The figure shows three views and two pictorial views of one solid part (mm, origin at its lowest corner). Answer the questions. A direction names the side the tool comes from. Coordinates: 2 decimals unless noted, no trailing zeros. Loops run counter-clockwise (first coordinate to the right, second up) from the corner with the lowest first, then second, coordinate; pieces in that order, holes last. Notation, with made-up numbers: (19, 3.25) - (51, 3.25) arc R28 ccw to (51, 34.25) - close; hole circle Ø7 at (35, 26.25). An arc over 180 degrees is marked (long way). One line per question, with ' | ' between items.
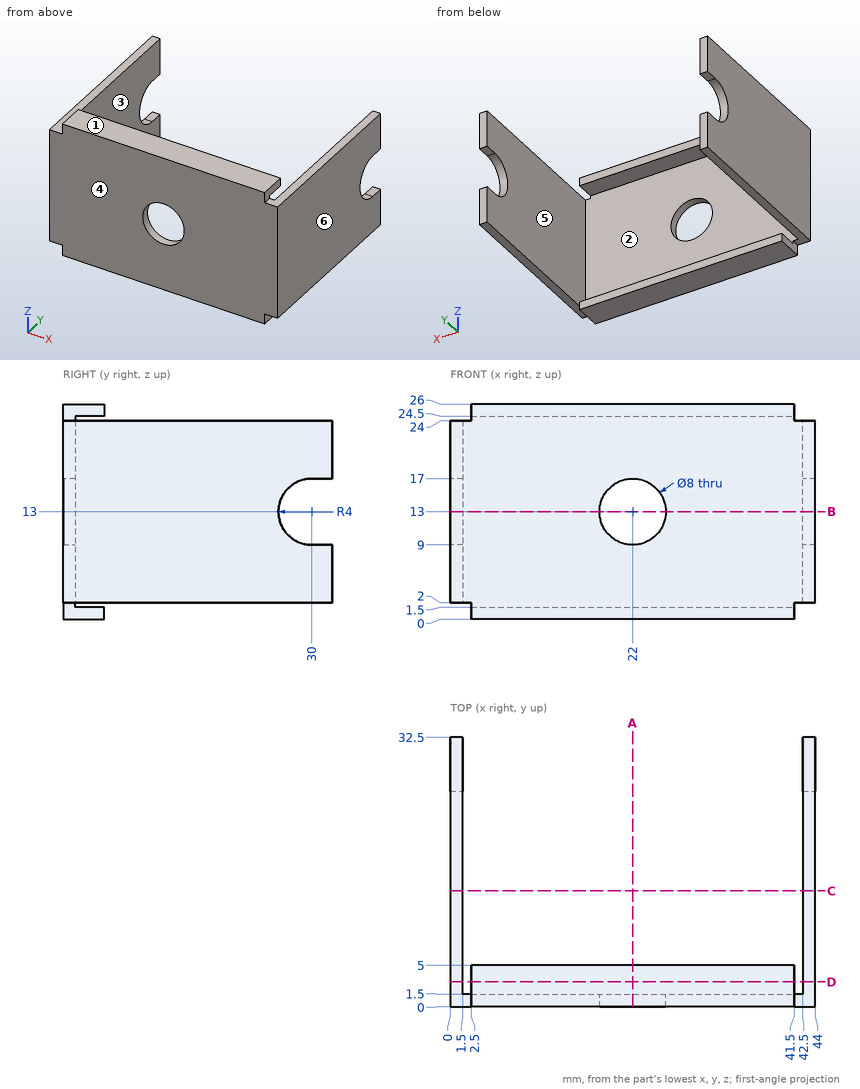
Item 1: Find section D-D, the plane y = 3. Write down the section's boundary in (x, z), plus the area to 3 significant figures.
Taken from the geometry:
outline: (0, 2) - (1.5, 2) - (1.5, 24) - (0, 24) - close; (2.5, 0) - (41.5, 0) - (41.5, 1.5) - (2.5, 1.5) - close; (2.5, 24.5) - (41.5, 24.5) - (41.5, 26) - (2.5, 26) - close; (42.5, 2) - (44, 2) - (44, 24) - (42.5, 24) - close | area: 183 mm2
Item 2: Find section C-C, the plane y = 14. Write down the section's boundary in (x, z).
Taken from the geometry:
outline: (0, 2) - (1.5, 2) - (1.5, 24) - (0, 24) - close; (42.5, 2) - (44, 2) - (44, 24) - (42.5, 24) - close
Item 3: Find section B-B, the plane z = 13. Write down the section's boundary in (x, y), plus the area to 4 significant figures.
Taken from the geometry:
outline: (0, 0) - (18, 0) - (18, 1.5) - (1.5, 1.5) - (1.5, 26) - (0, 26) - close; (26, 0) - (44, 0) - (44, 26) - (42.5, 26) - (42.5, 1.5) - (26, 1.5) - close | area: 127.5 mm2
Item 4: Each of these flat-tipped pins is pushed along its axis until it touches: pin 1 Ø1.6 at (x, z) = (26, 0.5) entering from +Y; pin 2 Ø1.2 at (x, y) = (42, 16.5) entering from +Z; pin 3 Ø1 at (y, z) = (3, 25) entering from -X. Where does it stop, or does it pass through?
Taken from the geometry:
pin 1: stops at y = 5 | pin 2: stops at z = 24 | pin 3: stops at x = 2.5
Item 5: Find the intervals of material crossed by line 1 (X direction, y = 1.1, z = 13); line 2 (X direction, y = 29, z = 21.25); line 3 (Y direction, x = 10.5, z = 9), in increasing order. Write a range as [from, to].
Taken from the geometry:
line 1: x = [0, 18], [26, 44] | line 2: x = [0, 1.5], [42.5, 44] | line 3: y = [0, 1.5]
Item 6: Find section A-A, the plane x = 22. Write down the section's boundary in (y, z).
Taken from the geometry:
outline: (0, 0) - (5, 0) - (5, 1.5) - (1.5, 1.5) - (1.5, 9) - (0, 9) - close; (0, 17) - (1.5, 17) - (1.5, 24.5) - (5, 24.5) - (5, 26) - (0, 26) - close
Item 7: Which of the six approach directions +Z, -Z, +X, -X, +Y, -Y give full straight-line access (tool end or side, diameter ignored) to the marked faces 1 and 2?
Taken from the geometry:
face 1: +Z, +X, -X, +Y, -Y | face 2: +Y
Item 8: The mould has two halves that part along X. Classify the marked faces 3, 4, 5 and 6: pulls with the +X half, pulls with the -X half, needs draft (parallel to the pull), parting line crosses it, or undercut.
Taken from the geometry:
face 3: undercut | face 4: needs draft | face 5: undercut | face 6: pulls with the +X half
